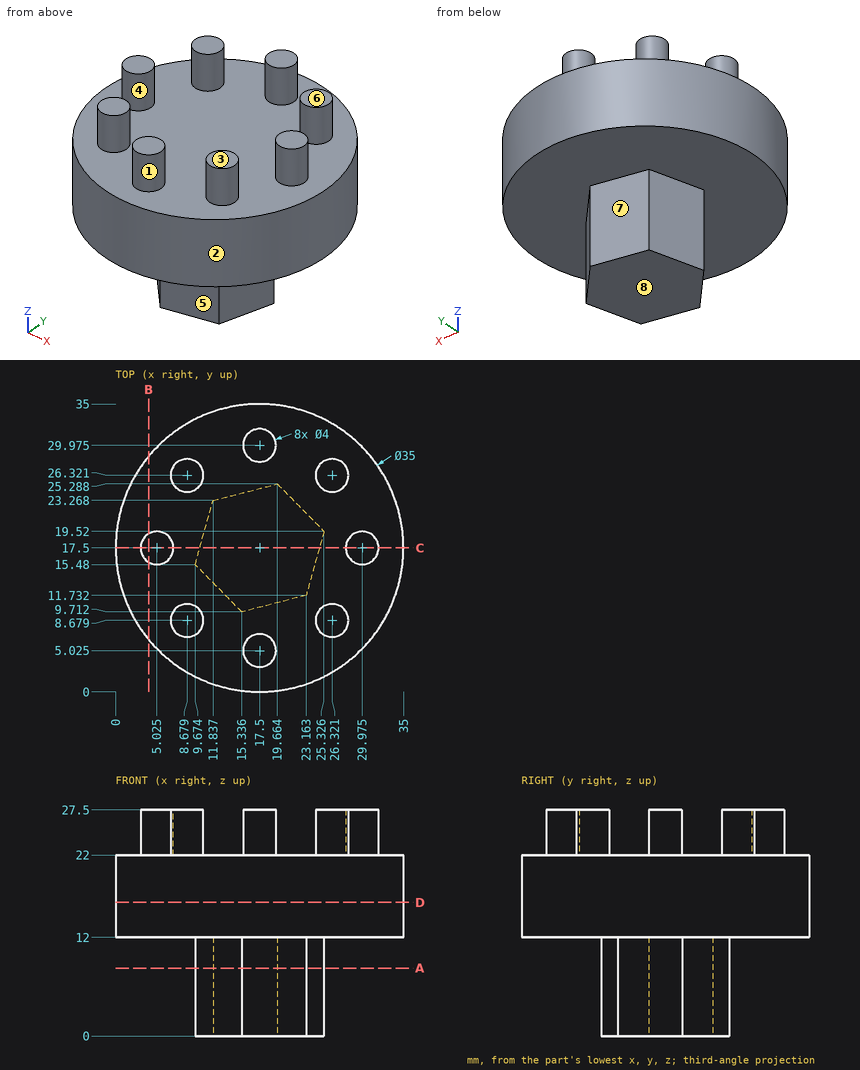
Study the drawing (mm; zero at the part's minimum x, y, z) and answer. A direction names the side the tool comes from. Give positions to 0.01 mm unless a question says otherwise; leave off trailing zeros. Order: outer loops, then holes, each group sorted by start corner. A loop starts at its lowest first (then second) coordinate and runs counter-clockwise, first axis right, second up. Notation, with made-up numbers: (65.25, 86.25) - (92.25, 86.25) arc R14 cw to (92.25, 94.25) - close; hole circle Ø9 at (80.25, 89). An arc over 180 degrees is marked (long way). Answer as CSV lines item,"result". Start each with the question number.
Q1. Given pin 1 Ø8 at (x, z) = (7.5, 22) entering from +Y; pin 2 Ø6 at (x, z) = (9.5, 11.5) entering from -Y; pin 3 Ø10 at (y, z) = (24, 17) entering from -X, each flat-ended and moving along its own axis, determine where each tip first touches the part or whether it passes through.
Q2. The part is cut by section C-C (y = 17.5). Write down the section's boundary in (x, z) (1 decimal).
Q3. The part is cut by section D-D (z = 16.25). Write down the section's boundary in (x, y), then the cut area to 3 significant figures.
Q4. The part is cut by section A-A (z = 8.25). Write down the section's boundary in (x, y), then the cut area to 3 significant figures.
Q5. The part is cut by section B-B (x = 4). Write down the section's boundary in (y, z) (1 decimal).
Q6. For the marked faces 4, 5, 6, 7 and 8, determine the directions among +Z, -Z, +X, -X, +Y, -Y from which every point of the face is accessible in a straight line to the end or side of a thin tool.
Q7. The mould has two halves that part along Y. Classify the marked faces 1, 2 and 3: +Y half, -Y half, draft (parallel to the pull), parting line (faces both ways), or undercut.
Q8. Find the intervals of material crossed by L1, parallel to Y at x = 17.5, z = 26.25 (1 decimal); L2, parallel to Z at x = 27.5, y = 31; L3, parallel to Z at x = 21, y = 16, in increasing order. Write a range as [from, to].
Check result:
1,pin 1,"stops at y = 33.94"
1,pin 2,"stops at y = 0.74"
1,pin 3,"stops at x = 0.06"
2,outline,"(0, 12) - (10.2, 12) - (10.2, 0) - (24.8, 0) - (24.8, 12) - (35, 12) - (35, 22) - (32, 22) - (32, 27.5) - (28, 27.5) - (28, 22) - (7, 22) - (7, 27.5) - (3, 27.5) - (3, 22) - (0, 22) - close"
3,outline,"circle Ø35 at (17.5, 17.5)"
3,area,"962 mm²"
4,outline,"(9.67, 15.48) - (15.34, 9.71) - (23.16, 11.73) - (25.33, 19.52) - (19.66, 25.29) - (11.84, 23.27) - close"
4,area,"170 mm²"
5,outline,"(6.4, 12) - (28.6, 12) - (28.6, 22) - (19.2, 22) - (19.2, 27.5) - (15.8, 27.5) - (15.8, 22) - (6.4, 22) - close"
6,face 4,"+Z"
6,face 5,"-Z, +X, -Y"
6,face 6,"+Z, +X, -X, +Y, -Y"
6,face 7,"-Z, -X, +Y"
6,face 8,"-Z, +X, -X, +Y, -Y"
7,face 1,"undercut"
7,face 2,"parting line"
7,face 3,"draft"
8,L1,"y = [3, 7], [28, 32]"
8,L2,"z = [12, 22]"
8,L3,"z = [0, 22]"
